Design review of the part built by this model. Coordinates are the model's own, in mm. Face numbers are marked on the shaded views. A direction names the side the tool comes from. Round coordinates to 2 decimals unless told otherwise and drop trailing zeros. Loops run counter-clockwise (first coordinate to the right, second up) from the corner with the lowest first, then second, coordinate; pieces in that order, holes last. Notation, with made-up numbers: M 9.25,70.5 L 34.25,70.5 A14 ccw 34.25,92.5 Z; hole C -21.75,72 d4. An arc over 180 degrees is marked long. Use a Markdown table: item, result.
from build123d import *

# Parameters (mm, degrees)
EXTRUDE_1_DEPTH          = 508
CUT_EXTRUDE_1_DEPTH      = 1048.268828907
CUT_EXTRUDE_1_DEPTH_BACK = 1048.268828907
CUT_EXTRUDE_2_DEPTH      = 1048.268828907
CUT_EXTRUDE_2_DEPTH_BACK = 1048.268828907
CUT_EXTRUDE_3_DEPTH      = 1048.268828907
CUT_EXTRUDE_3_DEPTH_BACK = 1048.268828907
SKETCH_5_R               = 254


with BuildPart() as part:
    # 草图2 → 凸台-拉伸1 (new, symmetric)
    with BuildSketch(Plane(origin=(0, 0, 0), x_dir=(0, 0, -1), z_dir=(1, 0, 0))):
        Polygon((0, 508), (762, 508), (762, -508), (-762, -508), (-762, 0), (0, -5.276054191), align=None)
    extrude(amount=EXTRUDE_1_DEPTH, both=True)

    # 草图3 → 切除-拉伸1 (cut, two sides: drawn at the far end of the back side and taken through both)
    with BuildSketch(Plane.XY.offset(-CUT_EXTRUDE_1_DEPTH_BACK)):
        with BuildLine():
            Line((-330.2, 508), (330.2, 508))
            ThreePointArc((330.2, 508), (0, 177.8), (-330.2, 508))
        make_face()
    extrude(amount=CUT_EXTRUDE_1_DEPTH + CUT_EXTRUDE_1_DEPTH_BACK, mode=Mode.SUBTRACT)

    # 草图4 → 切除-拉伸2 (cut, two sides: drawn at the far end of the back side and taken through both)
    with BuildSketch(Plane.XY.offset(-CUT_EXTRUDE_2_DEPTH_BACK)):
        Polygon((-406.4, -325.779762396), (406.4, -325.779762396), (254, -508), (-254, -508), align=None)
    extrude(amount=CUT_EXTRUDE_2_DEPTH + CUT_EXTRUDE_2_DEPTH_BACK, mode=Mode.SUBTRACT)

    # 草图5 → 切除-拉伸3 (cut, two sides: drawn at the far end of the back side and taken through both)
    with BuildSketch(Plane(origin=(0, 0, 0), x_dir=(1, 0, 0), z_dir=(0, 1, 0)).offset(-CUT_EXTRUDE_3_DEPTH_BACK)):
        with Locations(Location((0, -392.691654486, 0), (0, 0, 270))):
            Circle(SKETCH_5_R)
    extrude(amount=CUT_EXTRUDE_3_DEPTH + CUT_EXTRUDE_3_DEPTH_BACK, mode=Mode.SUBTRACT)


solid = part.part
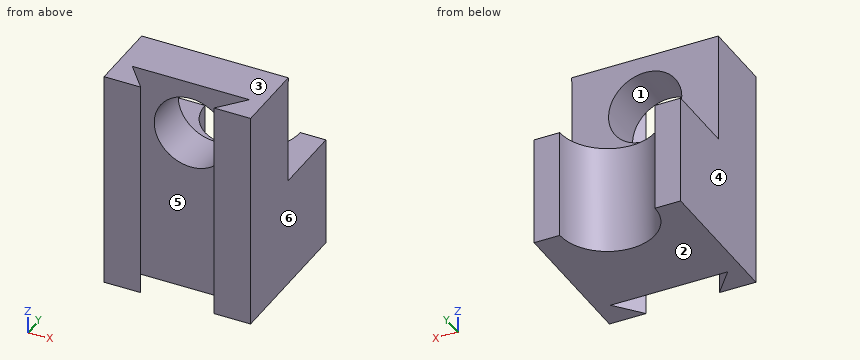
1. Insertion check: pin 1 (2 mm diameter, centred on x = -222.5, z = 532, fed in from -Y). The pin has a flat end and moves straight along its axis. Give the tip position at first contact, or say it passes through.
Check values:
| item | result |
|---|---|
| pin 1 | stops at y = -325.78 |
2. Machinability: for the marked faces 5 and 6, which of the approach directions +Z, -Z, +X, -X, +Y, -Y give a long, thin tool a straight path to every point of the face, cutting with its end or side? Answer none if there is none.
Check values:
| item | result |
|---|---|
| face 5 | +Z, -Z |
| face 6 | +Z, -Z, +X, +Y, -Y |
3. Take a section at A-A on x = -161.5. Give the boundary of the cut face in (y, z), and give its area (3 significant figures).
Check values:
| item | result |
|---|---|
| outline | M -325.78,-762 L 219.99,-762 L 219.99,0 L -5.28,0 L -3.91,196.65 L -325.78,196.65 Z; M -325.78,588.74 L -1.2,588.74 L 0,762 L -325.78,762 Z |
| area | 535,000 mm² |
4. Take a section at C-C on z = 424. Give the boundary of the cut face in (x, y).
Check values:
| item | result |
|---|---|
| outline | M -508,-508 L -254,-508 L -406.4,-325.78 L -252.06,-325.78 L -252.06,-2.34 L -508,-2.34 Z; M 252.06,-325.78 L 406.4,-325.78 L 254,-508 L 508,-508 L 508,-2.34 L 252.06,-2.34 Z |
5. Take a section at B-B on y = -434. Give the boundary of the cut face in (x, z), and give its area (3 significant figures).
Check values:
| item | result |
|---|---|
| outline | M -508,-762 L -315.89,-762 L -315.89,762 L -508,762 Z; M 315.89,-762 L 508,-762 L 508,762 L 315.89,762 Z |
| area | 586,000 mm² |
6. Take a section at D-D on y = -137. Give the boundary of the cut face in (x, z).
Check values:
| item | result |
|---|---|
| outline | M -508,-762 L 508,-762 L 508,762 L -508,762 Z; hole C 0,392.69 d508 |
7. Wall thickness on line 1 along Z through (x, y) = (0, -164); line 2 along Y through (x, z) = (-163, 0.5); line 3 along X through (y, z) = (-331, 521): over which ranges is each line inside the solid? List them lowest first. Write a range as from..to.
Check values:
| item | result |
|---|---|
| line 1 | z = -762..138.69, 646.69..762 |
| line 2 | y = -325.78..-5.27 |
| line 3 | x = -508..-402.03, 402.03..508 |
8. The part is to be moulded in two halves that separate along Z. For the marked faces 1, 2, 3 and 4, say which applies: pulls with the +Z half, pulls with the -Z half, needs draft (parallel to the pull), parting line crosses it, or undercut.
Check values:
| item | result |
|---|---|
| face 1 | undercut |
| face 2 | pulls with the -Z half |
| face 3 | pulls with the +Z half |
| face 4 | needs draft |
